For this review, take the finished solid that the model builds, in its own axes (mm). A direction names the side the tool comes from. Coordinates: 2 decimals unless noted, no trailing zeros. Loops run counter-clockwise (first coordinate to the right, second up) from the corner with the lowest first, then second, coordinate; pieces in that order, holes last.
1. Clearance check with flat-ended pins moving along their axes: P1, Ø2, axis at y = 12.5, z = 3, coming from the -X side; P2, Ø6, axis at x = 1.5, y = -5, coming from the +Z side; P3, Ø11, axis at y = 16, z = 1, coming from the +X side. State where each tip first meets the part, or that it passes through.
2. Machinability: for faces 1 (the face through (2.003, 12.599, 0.631)), 2 (the face through (-2.068, -17, 4)), 3 (the face through (0, 15, 6)), which of the approach directions +Z, -Z, +X, -X, +Y, -Y give a long, thin tool a straight path to every point of the face, cutting with its end or side? Answer none if there is none.
3. To check wall thickness, follow probe 1 along X at (y, z) = (13.5, 0); probe 2 along Y at (x, z) = (-1, 8). State the ranges of each line that lie inside material, in increasing order.
4. Mouldability with a two-part tool opening along Y and no side actions: class faces 4 (the face through (1.932, -18, 4)), 5 (the face through (0, -7.5, 4.2)), 6 (the face through (0, 15, -6)), 7 (the face through (-0.35, 4.46, 0.11)) as pulls with the +Y half, pulls with the -Y half, needs draft (parallel to the pull), parting line crosses it, or undercut.
5. Take a section at B-B, the plane x = -8. State the section outline as (y, z) points, then the cut area to 3 significant figures.
6. Take a section at A-A, the plane y = -17.5. State the section outline as (x, z) points, then the cut area to 3 significant figures.
7. Take a section at C-C, the plane y = -5. State the section outline as (x, z) points, then the cut area to 3 significant figures.
```python
from build123d import *

# Parameters (mm, degrees)
F0_R      = 5.5
F1_DEPTH  = 35
F2_R      = 10
F3_DEPTH  = 10
F4_W      = 12
F4_H      = 12
F5_DEPTH  = 9.9
F7_D      = 4.2
F7_DEPTH  = 14.4
F7_TIP    = 1.2618073
F10_DEPTH = 25
F11_R     = 1


with BuildPart() as f1:
    # F0 (on Front) → F1 (new body)
    with BuildSketch(Plane.XZ):
        Circle(F0_R)
    extrude(amount=F1_DEPTH)

    # F2 (on Front) → F3 (join)
    with BuildSketch(Plane.XZ):
        Circle(F2_R)
    extrude(amount=-F3_DEPTH)

    # F4 (on face) → F5 (join)
    with BuildSketch(Plane(origin=(0, 10, 0), x_dir=(-1, 0, 0), z_dir=(0, 1, 0))):
        Rectangle(F4_W, F4_H)
    extrude(amount=F5_DEPTH)

    # F7
    with Locations(Plane(origin=(0, 19.9, 0), x_dir=(-1, 0, 0), z_dir=(0, 1, 0))):
        with Locations((0, 0)):
            Hole(F7_D / 2, depth=F7_DEPTH)
            with Locations((0, 0, -(F7_DEPTH + F7_TIP / 2))):  # 118° drill point
                Cone(0, F7_D / 2, F7_TIP, mode=Mode.SUBTRACT)

    # F9 (on offset) → F10 (cut)
    with BuildSketch(Plane.XY.offset(3)):
        with BuildLine():
            ThreePointArc((1.9320917986, -9.4997572851), (-0.0679082014, -7.4997572851), (-2.0679082014, -9.4997572851))
            Line((-2.0679082014, -9.4997572851), (-2.0679082014, -25.4997572851))
            ThreePointArc((-2.0679082014, -25.4997572851), (-0.0679082014, -27.4997572851), (1.9320917986, -25.4997572851))
            Line((1.9320917986, -25.4997572851), (1.9320917986, -9.4997572851))
        make_face()
    extrude(amount=F10_DEPTH, mode=Mode.SUBTRACT)

    # F11
    f11_edges = [f1.edges().sort_by_distance(p)[0] for p in [
        (-5.5, -35, 0),
    ]]
    fillet(f11_edges, radius=F11_R)


solid = f1.part
```
Results list:
1. P1: stops at x = -6
1. P2: stops at z = 5.5
1. P3: stops at x = 6
2. face 1: +Y
2. face 2: +Z
2. face 3: +Z, +X, -X, +Y
3. probe 1: x = -6 to -2.1, 2.1 to 6
3. probe 2: y = 0 to 10
4. face 4: undercut
4. face 5: undercut
4. face 6: needs draft
4. face 7: pulls with the +Y half
5. outline: (0, -6) - (10, -6) - (10, 6) - (0, 6) - close
5. area: 120 mm2
6. outline: (-2.07, 3) - (-2.07, 5.1) arc R5.5 ccw (long way) to (1.93, 5.15) - (1.93, 3) - close
6. area: 85.5 mm2
7. outline: circle Ø11 at (0, 0)
7. area: 95.0 mm2
